Could you check a few things on this drawing? It's one solid part, dimensions in mm from its lowest x, y, z. A direction names the side the tool comes from. Give positions to 0.01 mm unless a question says otherwise; leave off trailing zeros. Order: outer loops, then holes, each group sorted by start corner. A loop starts at its lowest first (then second) coordinate and runs counter-clockwise, first axis right, second up. Notation, with made-up numbers: M 26.25,35 L 59.25,35 A15 cw 59.25,43 Z; hole C -38,-36.5 d5. An arc over 180 degrees is marked long. Use one line per item in the form item = value.
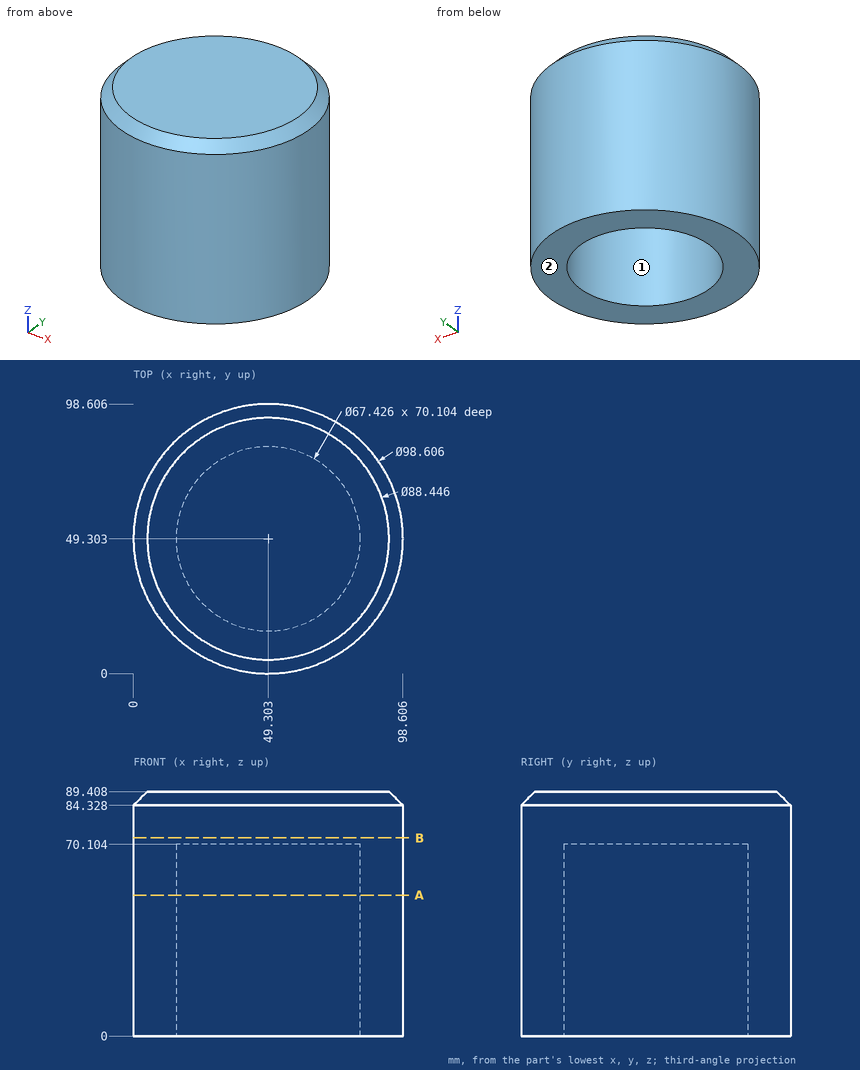
Q1. I want a section at A-A on z = 51.5. Write out the boundary of the cut face in (x, y).
Found:
outline = C 49.3,49.3 d98.61; hole C 49.3,49.3 d67.43
Q2. I want a section at B-B on z = 72.5. Write out the boundary of the cut face in (x, y).
Found:
outline = C 49.3,49.3 d98.61
Q3. I need wall thicknesses on L1, parallel to Y at x = 50, z = 44 (1 decimal); L2, parallel to Z at x = 52.5, y = 54.5; L3, parallel to X at y = 64, z = 55.5 (1 decimal). Which ranges of each line are inside material? Lowest first, please.
Found:
L1 = 0 to 15.6, 83 to 98.6
L2 = 70.1 to 89.41
L3 = 2.2 to 19, 79.6 to 96.4
Q4. On a 3-axis mill with a long thin cutter (end or side, diameter ignored), from which of +Z, -Z, +X, -X, +Y, -Y can I reach the whole of each face in a straight line? I mean the marked faces 1 and 2. Say none if no direction works.
Found:
face_1 = -Z
face_2 = -Z, +X, -X, +Y, -Y
Q5. I'm going to push flat-ended pins straight in: pin 1 Ø2 at (y, z) = (56, 14.5) entering from -X; pin 2 Ø10 at (x, z) = (44, 72) entering from -Y; pin 3 Ø1 at (y, z) = (50, 56) entering from +X. Where does each tip first touch, or does it pass through?
Found:
pin_1 = 0.33
pin_2 = 0
pin_3 = 98.61
